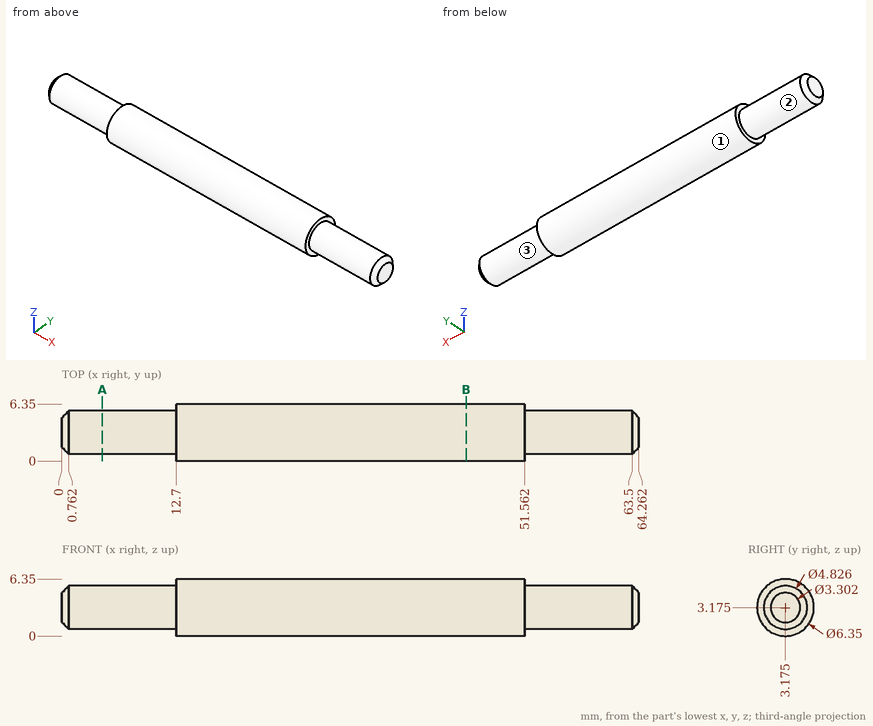
Source: three-view drawing plus pictorial views. Frame: mm from the lowest corner of the part. A direction names the side the tool comes from. Give positions to 0.01 mm unless a question says otherwise; leave off trailing zeros. Order: outer loops, then holes, each group sorted by start corner. A loop starts at its lowest first (then second) coordinate and runs counter-clockwise, first axis right, second up. Notation, with made-up numbers: M 25,10.5 L 33,10.5 A27 cw 33,40.5 Z; hole C -29,-10 d1. An arc over 180 degrees is marked long. One line per question, with ' | ' between items. Start each with the question number.
1. Material intervals for probe 1 along X at (y, z) = (5.5, 5); probe 2 along Y at (x, z) = (30.5, 3); probe 3 along Y at (x, z) = (29, 0.5), sorted ascending. Write a range as [from, to].
2. Section query B-B (x = 45). Return the cut outline in (y, z) (3 decimals), and give its area (3 significant figures).
3. Section query A-A (x = 4.5). Return the cut outline in (y, z) (3 decimals).
4. Access query for the marked faces 1, 2 and 3. Directions: +Z, -Z, +X, -X, +Y, -Y. A direction counts if a zero-diameter tool reaches every point of the face in a straight line with its end or side. Return the directions, or none.
Here are the results:
1) probe 1: [12.7, 51.56] | probe 2: [0, 6.35] | probe 3: [1.46, 4.89]
2) outline: C 3.175,3.175 d6.35 | area: 31.7 mm²
3) outline: C 3.175,3.175 d4.826
4) face 1: +X, -X | face 2: -X | face 3: +X
